Here's how the part is built. I have some questions about the finished solid (model axes, mm). A direction names the side the tool comes from. Give positions to 0.01 mm unless a question says otherwise; leave off trailing zeros. Order: outer loops, then holes, each group sorted by start corner. A loop starts at its lowest first (then second) coordinate and runs counter-clockwise, first axis right, second up. Notation, with made-up numbers: M 67,70 L 80,70 A19 cw 80,87 Z; hole C 61,33.25 d5. An arc over 180 degrees is marked long. One line per item, written item: value. Start each with the question number.
from build123d import *

# Parameters (mm, degrees)
F0_W         = 21.59
F0_H         = 62.21
F1_DEPTH     = 1.63
F4_DEPTH     = 12.34
F5_DEPTH     = 7.5
F2_R         = 1.25
F6_DEPTH     = 25
F7_SIZE      = 2
F8_R         = 1.2071067812
F10_DEPTH    = 8.23
F12_DEPTH    = 8.23
F13_T1_DEPTH = 10.2873463904
F14_W        = 7.51
F14_H        = 2.83
F14_H_2      = 5.48
F15_DEPTH    = 8.23


# Not quite as in the source:
# - a fillet or chamfer that OpenCascade refuses, or shapes differently, is made with other operations: its cross-section is extruded or revolved along the edge and cut away or added


with BuildPart() as f1:
    # F0 (on Top) → F1 (new body)
    with BuildSketch(Plane.XY):
        Rectangle(F0_W, F0_H)
    extrude(amount=F1_DEPTH)

    # F3 (on face) → F4 (join)
    with BuildSketch(Plane.XY.offset(1.63)):
        with BuildLine():
            ThreePointArc((10.7950629295, 14.605), (9.5971296646, 17.4970667351), (6.7050629295, 18.695))
            ThreePointArc((6.7050629295, 18.695), (2.6150629295, 14.605), (6.7050629295, 10.515))
            ThreePointArc((6.7050629295, 10.515), (9.5971296646, 11.7129332649), (10.7950629295, 14.605))
        make_face()
    extrude(amount=F4_DEPTH)

    # F3 (on face) → F5 (join)
    with BuildSketch(Plane.XY.offset(1.63)):
        Polygon((10.0900629295, -0.525), (6.7050629295, -0.525), (3.3200629295, -0.525), (3.3200629295, -7.975), (10.0900629295, -7.975), align=None)
    extrude(amount=F5_DEPTH)

    # F2 (on face) → F6 (cut)
    with BuildSketch(Plane.XY.offset(1.63)):
        with BuildLine():
            ThreePointArc((7.675, 29.005), (6.7911165235, 26.8711165235), (8.925, 27.755))
            Line((8.925, 27.755), (7.675, 27.755))
            Line((7.675, 27.755), (7.675, 29.005))
        make_face()
        with BuildLine():
            Line((7.675, 27.755), (8.925, 27.755))
            ThreePointArc((8.925, 27.755), (8.5588834765, 28.6388834765), (7.675, 29.005))
            Line((7.675, 29.005), (7.675, 27.755))
        make_face()
        with Locations((-7.675, 27.755)):
            Circle(F2_R)
        with Locations((-7.675, -27.755)):
            Circle(F2_R)
        with Locations((7.675, -27.755)):
            Circle(F2_R)
    extrude(amount=-F6_DEPTH, mode=Mode.SUBTRACT)

    # F7
    f7_edges = [f1.edges().sort_by_distance(p)[0] for p in [
        (3.320063, -4.25, 9.13),
        (10.090063, -4.25, 9.13),
    ]]
    chamfer(f7_edges, length=F7_SIZE)

    # F8
    f8_edges = [f1.edges().sort_by_distance(p)[0] for p in [
        (6.705063, 18.695, 13.97),
    ]]
    fillet(f8_edges, radius=F8_R)

    # F9 (on face) → F10 (join)
    with BuildSketch(Plane.XY.offset(1.63)):
        Polygon((-10.795, 25.38), (-10.795, 0), (-10.795, -25.38), (-3.285, -25.38), (-3.285, 25.38), align=None)
    extrude(amount=F10_DEPTH)

    # F11 (on face) → F12 (join)
    with BuildSketch(Plane.XY.offset(1.63)):
        with BuildLine():
            Line((7.485, 31.105), (0, 31.105))
            Line((0, 31.105), (-7.485, 31.105))
            Line((-7.485, 31.105), (-7.485, 28.9904756169))
            ThreePointArc((-7.485, 28.9904756169), (-7.0487343616, 28.8368000509), (-6.6982195743, 28.535))
            Line((-6.6982195743, 28.535), (6.6982195743, 28.535))
            ThreePointArc((6.6982195743, 28.535), (7.0487343616, 28.8368000509), (7.485, 28.9904756169))
            Line((7.485, 28.9904756169), (7.485, 31.105))
        make_face()
        with BuildLine():
            Line((7.485, 28.535), (7.485, 28.9904756169))
            ThreePointArc((7.485, 28.9904756169), (7.0487343616, 28.8368000509), (6.6982195743, 28.535))
            Line((6.6982195743, 28.535), (7.485, 28.535))
        make_face()
        with BuildLine():
            ThreePointArc((-6.6982195743, 28.535), (-7.0487343616, 28.8368000509), (-7.485, 28.9904756169))
            Line((-7.485, 28.9904756169), (-7.485, 28.535))
            Line((-7.485, 28.535), (-6.6982195743, 28.535))
        make_face()
        with BuildLine():
            Line((0, -31.105), (7.485, -31.105))
            Line((7.485, -31.105), (7.485, -28.9904756169))
            ThreePointArc((7.485, -28.9904756169), (7.0487343616, -28.8368000509), (6.6982195743, -28.535))
            Line((6.6982195743, -28.535), (-6.6982195743, -28.535))
            ThreePointArc((-6.6982195743, -28.535), (-7.0487343616, -28.8368000509), (-7.485, -28.9904756169))
            Line((-7.485, -28.9904756169), (-7.485, -31.105))
            Line((-7.485, -31.105), (0, -31.105))
        make_face()
        with BuildLine():
            ThreePointArc((6.6982195743, -28.535), (7.0487343616, -28.8368000509), (7.485, -28.9904756169))
            Line((7.485, -28.9904756169), (7.485, -28.535))
            Line((7.485, -28.535), (6.6982195743, -28.535))
        make_face()
        with BuildLine():
            Line((-7.485, -28.535), (-7.485, -28.9904756169))
            ThreePointArc((-7.485, -28.9904756169), (-7.0487343616, -28.8368000509), (-6.6982195743, -28.535))
            Line((-6.6982195743, -28.535), (-7.485, -28.535))
        make_face()
    extrude(amount=F12_DEPTH)

    # F13: chamfer of 0.8 on 4 edges, made by hand

    # F13_s2 → F13_t1 (cut)
    with BuildSketch(Plane.XY.offset(1.63)):
        Polygon((-7.485, 29.335), (-6.685, 28.535), (-7.485, 28.535), align=None)
        Polygon((6.685, 28.535), (7.485, 29.335), (7.485, 28.535), align=None)
        Polygon((-6.685, -28.535), (-7.485, -29.335), (-7.485, -28.535), align=None)
        Polygon((7.485, -29.335), (6.685, -28.535), (7.485, -28.535), align=None)
    extrude(amount=F13_T1_DEPTH, mode=Mode.SUBTRACT)

    # F14 (on face) → F15 (cut)
    with BuildSketch(Plane.XY.offset(9.86)):
        with Locations((-7.04, 14.185)):
            Rectangle(F14_W, F14_H)
        with Locations((-7.04, 0.25)):
            Rectangle(F14_W, F14_H_2)
        with Locations((-7.04, -13.685)):
            Rectangle(F14_W, F14_H)
    extrude(amount=-F15_DEPTH, mode=Mode.SUBTRACT)


solid = f1.part
Item 1: Please list where these lines run through material, in increasing order: probe 1 along Y at (x, z) = (-6.25, 2.25) (3 decimals); probe 2 along Y at (x, z) = (7.25, 3.5) (3 decimals); probe 3 along Y at (x, z) = (5.75, 6.25) (3 decimals). Write a range as [from, to].
Item 2: We'd pull the mould along Y, two halves only. Please class faces 1 (the face through (-3.285, 20, 6)), 2 (the face through (10.795, 0, 1)): +Y half, -Y half, draft (parallel to the pull), parting line (faces both ways), or undercut.
Item 3: I want a section at B-B on x = -0.75. Write out the boundary of the cut face in (y, z) (3 decimals), plus the area to 3 significant figures.
Item 4: I want a section at D-D on z = 11.5. Write out the boundary of the cut face in (x, y) (3 decimals), plus the area to 3 significant figures.
Item 5: Will these pins go through, and if not, where does the flat tip stop? P1, Ø5, axis at x = -2, y = -5, coming from the +Z side; P2, Ø1.9, axis at y = 30.5, z = 5.5, coming from the -X side (3 decimals); P3, Ø1, axis at y = 23, z = 7, coming from the +X side (3 decimals).
Item 6: I want a section at C-C on z = 6.5. Count the separate pieces of the cut face and the enclosed holes in it, plus the area to 3 significant figures.
Item 7: For faces 3 (the face through (-7, 21, 9.86)), 4 (the face through (0, -28.535, 6)), 5 (the face through (4.33, -4.2, 8.14)), which set-ups out of +Z, -Z, +X, -X, +Y, -Y let a thin tool reach every point of the face, with its end or its side?
Item 8: I want a section at A-A on y = -6.5. Write out the boundary of the cut face in (x, z) (3 decimals).
Answer below:
1. probe 1: y = [-31.105, -28.535], [-25.38, -15.1], [-12.27, -2.49], [2.99, 12.77], [15.6, 25.38], [28.535, 31.105]
1. probe 2: y = [-31.105, -29.1], [-7.975, -0.525], [10.551, 18.659], [29.1, 31.105]
1. probe 3: y = [-31.105, -28.535], [-7.975, -0.525], [10.628, 18.582], [28.535, 31.105]
2. face 1: undercut
2. face 2: draft
3. outline: M -31.105,0 L 31.105,0 L 31.105,9.86 L 28.535,9.86 L 28.535,1.63 L -28.535,1.63 L -28.535,9.86 L -31.105,9.86 Z
3. area: 144 mm²
4. outline: C 6.705,14.605 d8.18
4. area: 52.6 mm²
5. P1: stops at z = 9.86
5. P2: stops at x = -7.485
5. P3: stops at x = -3.285
6. separate pieces: 8
6. enclosed holes: 0
6. area: 476 mm²
7. face 3: +Z, -X, +Y, -Y
7. face 4: +Z, +X, -X
7. face 5: +Z
8. outline: M -10.795,0 L 10.795,0 L 10.795,1.63 L 10.09,1.63 L 10.09,7.13 L 8.09,9.13 L 5.32,9.13 L 3.32,7.13 L 3.32,1.63 L -3.285,1.63 L -3.285,9.86 L -10.795,9.86 Z
